Part model, mm, in its own coordinate system. A direction names the side the tool comes from. Coordinates: 2 decimals unless noted, no trailing zeros. Order: outer loops, then holes, each group sorted by start corner. A loop starts at its lowest first (then second) coordinate and runs counter-clockwise, first axis right, second up. Notation, with made-up numbers: (32, -39.75) - (40, -39.75) arc R12 ccw to (40, -35.75) - close; hole circle Ø5 at (-9.5, 19.5). An arc over 180 degrees is marked (long way). Use a Markdown table: item, result. Add a question column.
1) Tool access for faces 5 (the face through (-15, 37, 12.7)), 6 (the face through (-15, 25, 0)): list every direction of +Z, -Z, +X, -X, +Y, -Y with a clear straight run to the whole face (end or side of a thin tool).
2) Saw through at A-A on x = 24.5. List the corners of the cut face in (y, z), then the cut area to 3 significant figures.
3) Wall check: L1, parallel to Y at x = -21, z = 35; L2, parallel to Y at x = 35, z = 12.5 (3 decimals); L3, parallel to X at y = -7.5, z = 40. Give the ranges that are in metal, low to high. Write a range as [from, to].
4) Drop flat-ended pins along their axis: P1, Ø12, axis at x = 39.93, y = 38.99, coming from the +Z side; P2, Ø3, axis at x = 41.5, y = 41.5, coming from the +Z side. Give the stop position or say it passes through.
5) Saw through at C-C on z = 43.5. List the corners of the cut face in (x, y).
6) Saw through at D-D on x = -18. List the corners of the cut face in (y, z), then the cut area to 3 significant figures.
7) Saw through at B-B on y = 22.5. List the corners of the cut face in (x, z).
8) Two-plate mould, pull along Y, no slides. Class faces 1 (the face through (-14.842, 43.565, 31.483)), 2 (the face through (39.26, -33, 31.48)), 3 (the face through (-15, 25, 50.8)), 4 (the face through (12, -37.413, 25)): +Y half, -Y half, draft (parallel to the pull), parting line (faces both ways), or undercut.
Autodesk Inventor part; units mm, degrees
ref_plane "YZ Plane" through (0, 0, 0) normal (1, 0, 0) x (0, 1, 0)
ref_plane "XZ Plane" through (0, 0, 0) normal (0, 1, 0) x (-1, 0, 0)
ref_plane "XY Plane" through (0, 0, 0) normal (0, 0, 1) x (1, 0, 0)
sketch "Sketch1" plane through (0, 0, 0) normal (0, 0, 1) x (1, 0, 0)
  line L0 (-26.7465, 47.6774) -> (49.4535, 47.6774)
  line L1 (49.4535, 47.6774) -> (49.4535, -37.4126)
  line L2 (49.4535, -37.4126) -> (-26.7465, -37.4126)
  line L3 (-26.7465, -37.4126) -> (-26.7465, 47.6774)
  line L4 (-26.7465, 47.6774) -> (-9.2459, 47.6774)
  line L5 (49.4535, 47.6774) -> (31.9529, 47.6774)
  line L6 (49.4535, 47.6774) -> (49.4535, 41.683)
  line L7 (49.4535, -37.4126) -> (49.4535, -31.4182)
  circle A0 centre (11.3535, 5.1324) radius 31.75
  line L8 (-26.7465, 47.6774) -> (-17.2215, 47.6774)
  line L9 (49.4535, 47.6774) -> (39.9285, 47.6774)
  line L10 (-26.7465, -37.4126) -> (-26.7465, -27.8876)
  circle A1 centre (-17.2215, -27.8876) radius 2.7813
  circle A2 centre (39.9285, -27.8876) radius 2.7813
  circle A3 centre (39.9285, 38.9906) radius 2.7813
  line L11 (-26.7465, -27.8876) -> (-17.2215, -27.8876)
  circle A4 centre (-17.2215, 38.9906) radius 2.7813
  point P0 (0, 0)
  dimension "d0" = 76.2
  dimension "d1" = 85.09
  dimension "d2" = 17.5006
  dimension "d3" = 17.5006
  dimension "d4" = 5.9944
  dimension "d5" = 5.9944
  dimension "d25" = 63.5
  dimension "d26" = 9.525
  dimension "d30" = 9.525
  dimension "d31" = 5.5626
  dimension "d32" = 5.5626
  dimension "d45" = 5.5626
  dimension "d46" = 9.525
  dimension "d48" = 5.5626
extrude "Extrusion6" add sketch "Sketch1" along normal blind 12.7
sketch "Sketch4" plane through (0, 0, 12.7) normal (0, 0, 1) x (1, 0, 0)
  circle A0 centre (11.3535, 5.1324) radius 31.75
  circle A1 centre (-17.2215, 38.9906) radius 2.7813
  circle A2 centre (39.9285, -27.8876) radius 2.7813
  circle A3 centre (-17.2215, -27.8876) radius 2.7813
  circle A4 centre (39.9285, 38.9906) radius 2.7813
  line L0 (-26.7465, 47.6774) -> (49.4535, 47.6774)
  line L1 (-26.7465, -37.4126) -> (-26.7465, 47.6774)
  line L2 (-26.7465, -37.4126) -> (49.4535, -37.4126)
  line L3 (49.4535, -37.4126) -> (49.4535, 47.6774)
  line L4 (49.4535, 47.6774) -> (-26.7465, 47.6774)
  line L5 (-26.7465, 47.6774) -> (-26.7465, -37.4126)
  circle A5 centre (11.3535, 5.1324) radius 31.75
  circle A6 centre (-17.2215, -27.8876) radius 5.1562
  circle A7 centre (-17.2215, 38.9906) radius 5.1562
  circle A8 centre (39.9285, 38.9906) radius 5.1562
  circle A9 centre (39.9285, -27.8876) radius 5.1562
  point P0 (0, 0)
  dimension "d51" = 10.3124
  dimension "d52" = 10.3124
  dimension "d53" = 10.3124
  dimension "d54" = 10.3124
extrude "Extrusion7" add sketch "Sketch4" along normal blind 38.1 contours L0 L3 L2 L1
properties part number "glass socket"
Results are:
| question | item | result |
|---|---|---|
| 1 | face 5 | +Z |
| 1 | face 6 | -Z, +X, -X, +Y, -Y |
| 2 | outline | (-37.41, 0) - (-23.77, 0) - (-23.77, 50.8) - (-37.41, 50.8) - close; (34.03, 0) - (47.68, 0) - (47.68, 50.8) - (34.03, 50.8) - close |
| 2 | area | 1,390 mm2 |
| 3 | L1 | [-37.41, -31.4], [-24.38, 35.48], [42.5, 47.68] |
| 3 | L2 | [-37.413, -16.055], [26.32, 47.677] |
| 3 | L3 | [-26.75, -17.78], [40.48, 49.45] |
| 4 | P1 | z = 50.8 |
| 4 | P2 | z = 12.7 |
| 5 | outline | (-26.75, -37.41) - (49.45, -37.41) - (49.45, 47.68) - (-26.75, 47.68) - close; hole circle Ø10.31 at (-17.22, -27.89); hole circle Ø10.31 at (-17.22, 38.99); hole circle Ø63.5 at (11.35, 5.13); hole circle Ø10.31 at (39.93, -27.89); hole circle Ø10.31 at (39.93, 38.99) |
| 6 | outline | (-37.41, 0) - (-30.56, 0) - (-30.56, 12.7) - (-32.98, 12.7) - (-32.98, 50.8) - (-37.41, 50.8) - close; (-25.22, 0) - (-6.97, 0) - (-6.97, 50.8) - (-22.79, 50.8) - (-22.79, 12.7) - (-25.22, 12.7) - close; (17.23, 0) - (36.32, 0) - (36.32, 12.7) - (33.89, 12.7) - (33.89, 50.8) - (17.23, 50.8) - close; (41.66, 0) - (47.68, 0) - (47.68, 50.8) - (44.09, 50.8) - (44.09, 12.7) - (41.66, 12.7) - close |
| 6 | area | 2,180 mm2 |
| 7 | outline | (-26.75, 0) - (-15.23, 0) - (-15.23, 50.8) - (-26.75, 50.8) - close; (37.93, 0) - (49.45, 0) - (49.45, 50.8) - (37.93, 50.8) - close |
| 8 | face 1 | undercut |
| 8 | face 2 | undercut |
| 8 | face 3 | draft |
| 8 | face 4 | -Y half |
